from build123d import *

# Parameters (mm, degrees)
F0_W          = 55
F0_H          = 5
F1_DEPTH      = 5
F2_DEPTH      = 10
F2_DEPTH_BACK = 5
F4_D          = 3.2
F4_DEPTH      = 2.001


with BuildPart() as f1:
    # F0 (on Front) → F1 (new body)
    with BuildSketch(Plane.XZ):
        with Locations((29.5, 2.5)):
            Rectangle(F0_W, F0_H)
        Polygon((57, 5), (57, 0), (59, 0), (59, 10), (57, 10), align=None)
    extrude(amount=F1_DEPTH)

    # F0 (on Front) → F2 (join, two sides)
    with BuildSketch(Plane.XZ) as f2_sk:
        Polygon((0, 15), (0, 0), (2, 0), (2, 5), (2, 15), align=None)
    extrude(amount=F2_DEPTH)
    extrude(f2_sk.sketch, amount=-F2_DEPTH_BACK)

    # F4 (through all, one way)
    with BuildSketch(Plane.YZ.offset(2)):
        with Locations((-2.5, 10.4)):
            Circle(F4_D / 2)
    extrude(amount=-F4_DEPTH, mode=Mode.SUBTRACT)


solid = f1.part
Could you check a few things on this model? Use its own coordinates, in mm. A direction names the side the tool comes from. Coordinates: 2 decimals unless noted, no trailing zeros. Order: outer loops, then holes, each group sorted by start corner. A loop starts at its lowest first (then second) coordinate and runs counter-clockwise, first axis right, second up.
Q1. Thinking about a two-plate mould opening in X: for faces 6 (the flat face through (29, -2, 5)), 7 (the flat face through (0, -3, 8)), 8 (the flat face through (1, -3, 15)), which applies, released by +X, released by -X, zero draft, split by the parting line, or undercut?
Q2. Suppose I cut it at D-D on y = 1.25. Please give me the cut outline in (x, z).
Q3. Suppose I cut it at B-B on z = 6. Please give me the cut outline in (x, y).
Q4. Which directions (+Z, -Z, +X, -X, +Y, -Y) give clear straight access to the entire face, cutting with the end or side of a thin tool? Please do faces 1 (the flat face through (30, 0, 3)), 2 (the cylindrical face through (1.01, -2.85, 8.84)), 3 (the flat face through (58, -2, 10)), 4 (the flat face through (57, -2, 8)), 5 (the flat face through (30, -5, 2)).
Q5. Please list where these lines run through material, in increasing order: L1, parallel to Z at x = 1, y = -2.5; L2, parallel to X at y = -3.5, z = 7.5; L3, parallel to X at y = -1.5, z = 14.
Q6. Suppose I cut it at A-A on y = -2.5. Please give me the cut outline in (x, z).
Q7. Will these pins go through, and if not, where does the flat tip stop? pin 1 (8 mm diameter, centred on x = 9.5, y = -6.5, fed in from +Z); pin 2 (2 mm diameter, centred on y = 1.5, z = 7.5, fed in from +X); pin 3 (1.5 mm diameter, centred on x = 26, z = 2.5, fed in from +Y).
Q8. Suppose I cut it at C-C on z = 2.75. Please give me the cut outline in (x, y).
Answer:
1. face 6: undercut
1. face 7: released by -X
1. face 8: zero draft
2. outline: (0, 0) - (2, 0) - (2, 15) - (0, 15) - close
3. outline: (0, -10) - (2, -10) - (2, 5) - (0, 5) - close; (57, -5) - (59, -5) - (59, 0) - (57, 0) - close
4. face 1: +Z, -Z, +X, +Y
4. face 2: -X
4. face 3: +Z, +X, +Y, -Y
4. face 4: +Z, +Y, -Y
4. face 5: +Z, -Z, +X, -Y
5. L1: z = 0 to 8.8, 12 to 15
5. L2: x = 0 to 2, 57 to 59
5. L3: x = 0 to 2
6. outline: (0, 0) - (59, 0) - (59, 10) - (57, 10) - (57, 5) - (2, 5) - (2, 8.8) - (0, 8.8) - close; (0, 12) - (2, 12) - (2, 15) - (0, 15) - close
7. pin 1: stops at z = 5
7. pin 2: stops at x = 2
7. pin 3: stops at y = 0
8. outline: (0, -10) - (2, -10) - (2, -5) - (59, -5) - (59, 0) - (2, 0) - (2, 5) - (0, 5) - close
